```python
from build123d import *

# Parameters (mm, degrees)
PRUREZ_R                 = 5
SKICA3_R                 = 10
P_IDAT_VYSUNUT_M1_DEPTH  = 30
SKICA4_R                 = 2.5
ODEBRAT_VYSUNUT_M1_DEPTH = 156.515429595


with BuildPart() as part:
    # Táhnout po křivce1: sweep along a path in Draha
    with BuildLine(Plane.XY) as t_hnout_po_k_ivce1_path:
        Line((0, 0), (90.673846837, 0))
        ThreePointArc((90.673846837, 0), (99.126212072, -1.873844259), (105.994735699, -7.144247806))
        Line((105.994735699, -7.144247806), (141.954981559, -50))
    # Prurez → Táhnout po křivce1 (sweep)
    with BuildSketch(Plane(origin=(0, 0, 0), x_dir=(0, 0, -1), z_dir=(1, 0, 0))):
        Circle(PRUREZ_R)
    sweep(path=t_hnout_po_k_ivce1_path.line)

    # Skica3 → Přidat vysunutím1 (add)
    with BuildSketch(Plane.ZY):
        Circle(SKICA3_R)
    extrude(amount=-P_IDAT_VYSUNUT_M1_DEPTH)

    # Skica4 → Odebrat vysunutím1 (cut, through all)
    with BuildSketch(Plane.ZY):
        with Locations((0, -28)):
            Circle(SKICA4_R)
    extrude(amount=-ODEBRAT_VYSUNUT_M1_DEPTH, mode=Mode.SUBTRACT)


solid = part.part
```
The listing builds one solid part. Answer for the finished solid, in the listing's coordinates (mm). A direction names the side the tool comes from. Give positions to 0.01 mm unless a question says otherwise; leave off trailing zeros. Loops run counter-clockwise (first coordinate to the right, second up) from the corner with the lowest first, then second, coordinate; pieces in that order, holes last. Notation, with made-up numbers: (10, -23) - (39, -23) arc R16 cw to (39, -2) - close; hole circle Ø9 at (17, 70.5). An arc over 180 degrees is marked (long way). Answer as CSV lines item,"result". Start each with the question number.
Item 1: Each of these flat-tipped pins is pushed along its axis until it touches: pin 1 (6 mm diameter, centred on x = 101.5, z = -1, fed in from -Y); pin 2 (10 mm diameter, centred on x = 67, z = 7, fed in from +Y); pin 3 (3 mm diameter, centred on y = 3.5, z = 0.5, fed in from +X). Where does it stop, or does it pass through?
Item 2: A cutting plane is placed at D-D on z = 7.5. Determine the outline of the cut face in (x, y).
Item 3: The mould has two halves that part along Y. Classify faces 3 (the face through (30, -2, -5)), 4 (the face through (123.376, -27.249, 2.385)), 5 (the face through (14.79, -9.76, -2.17)): +Y half, -Y half, draft (parallel to the pull), parting line (faces both ways), or undercut.
Item 4: A cutting plane is placed at A-A on z = 0. Determine the outline of the cut face in (x, y), then the cut area to 3 significant figures.
Item 5: A cutting plane is placed at B-B on x = 86.5. Determine the outline of the cut face in (y, z), then the cut area to 3 significant figures.
Item 6: For faces 1 (the face through (142.009, -49.955, -0.07)), 2 (the face through (60.76, -4.88, 1.08)), determine the directions among +Z, -Z, +X, -X, +Y, -Y from which every point of the face is accessible in a straight line to the end or side of a thin tool.
Item 7: A cutting plane is placed at C-C on z = -6.5. Determine the outline of the cut face in (x, y).
Item 8: Find the intervals of material crossed by line 1 (X direction, y = 6, z = -5.75); line 2 (Z direction, x = 121, y = -28); line 3 (Z direction, x = 119.75, y = -28), in increasing order. Write a range as from..to.
Found:
1,pin 1,"stops at y = -13.05"
1,pin 2,"stops at y = 4.58"
1,pin 3,"stops at x = 102.51"
2,outline,"(0, -6.61) - (30, -6.61) - (30, 6.61) - (0, 6.61) - close"
3,face 3,"draft"
3,face 4,"undercut"
3,face 5,"parting line"
4,outline,"(0, -10) - (30, -10) - (30, -5) - (90.67, -5) arc R15 cw to (102.16, -10.36) - (114.87, -25.5) - (127.92, -25.5) - (109.82, -3.93) arc R25 ccw to (90.67, 5) - (30, 5) - (30, 10) - (0, 10) - close; (119.07, -30.5) - (138.12, -53.21) - (145.79, -46.79) - (132.12, -30.5) - close"
4,area,"1,880 mm^2"
5,outline,"circle Ø10 at (0, 0)"
5,area,"78.5 mm^2"
6,face 1,"+Z, -Z, +X, -Y"
6,face 2,"none"
7,outline,"(0, -7.6) - (30, -7.6) - (30, 7.6) - (0, 7.6) - close"
8,line 1,"x = 0..30"
8,line 2,"z = -4.62..-2.5, 2.5..4.62"
8,line 3,"z = -4.1..-2.5, 2.5..4.1"
